Autodesk Inventor part; units mm, degrees
ref_plane "YZ Plane" through (0, 0, 0) normal (1, 0, 0) x (0, 1, 0)
ref_plane "XZ Plane" through (0, 0, 0) normal (0, 1, 0) x (-1, 0, 0)
ref_plane "XY Plane" through (0, 0, 0) normal (0, 0, 1) x (1, 0, 0)
sketch "Sketch1" plane through (0, 0, 0) normal (0, 0, 1) x (1, 0, 0)
  line L0 (19.1414, -92.5) -> (-27.8586, -92.5) construction
  line L1 (0, 3) -> (19.1414, 3) construction
  line L2 (6.5333, -102.5) -> (6.5333, -92.5) construction
  line L3 (-26.1333, -92.5) -> (-26.1333, -102.5) construction
  line L4 (-26.1333, -92.5) -> (-20.6889, -92.5)
  line L5 (19.1414, 3) -> (-27.8586, 3)
  line L6 (-27.8586, 3) -> (-27.8586, -92.5)
  line L7 (-27.8586, -92.5) -> (-20.6889, -92.5)
  line L8 (19.1414, -92.5) -> (19.1414, 3)
  line L9 (-27.8586, 3) -> (19.1414, 3)
  line L10 (19.1414, 3) -> (19.1414, 8)
  line L11 (19.1414, 8) -> (-27.8586, 8)
  line L12 (-27.8586, 8) -> (-27.8586, 3)
  line L13 (-6.3, -92.5) -> (-6.3, -95.5)
  line L14 (-6.3, -95.5) -> (1.0889, -95.5)
  line L15 (1.0889, -95.5) -> (1.0889, -92.5)
  line L16 (-13.3, -92.5) -> (-13.3, -95.5)
  line L17 (-13.3, -95.5) -> (-20.6889, -95.5)
  line L18 (-20.6889, -95.5) -> (-20.6889, -92.5)
  line L19 (-8.3, -92.5) -> (-8.3, -90.5)
  line L20 (-8.3, -90.5) -> (-7.15, -90.5)
  line L21 (-7.15, -90.5) -> (-7.15, -88.1)
  line L22 (-7.15, -88.1) -> (-8.3, -88.1)
  line L23 (-8.3, -88.1) -> (-8.3, -87.5)
  line L24 (-8.3, -87.5) -> (-11.3, -87.5)
  line L25 (-11.3, -87.5) -> (-11.3, -88.1)
  line L26 (-11.3, -88.1) -> (-12.45, -88.1)
  line L27 (-12.45, -88.1) -> (-12.45, -90.5)
  line L28 (-12.45, -90.5) -> (-11.3, -90.5)
  line L29 (-11.3, -92.5) -> (-11.3, -90.5)
  line L30 (-8.3, -92.5) -> (-6.3, -92.5)
  line L31 (-13.3, -92.5) -> (-11.3, -92.5)
  line L32 (-9.8, -83.4221) -> (-9.8, -94.6081) construction
  line L33 (-13.3, -92.5) -> (-11.3, -92.5)
  line L34 (1.0889, -92.5) -> (19.1414, -92.5)
  dimension "d4" = 5
  dimension "d13" = 5.3
  dimension "d14" = 2.4
  dimension "d15" = 3
  dimension "d16" = 32.6667
  dimension "d18" = 5.4444
  dimension "d19" = 5.4444
  dimension "d20" = 21.7778
  dimension "d21" = 7
  dimension "d22" = 3
  dimension "d23" = 5
  dimension "d24" = 8
extrude "Extrusion1" add sketch "Sketch1" along normal blind 3
sketch "Sketch2" plane through (0, 0, 3) normal (0, 0, 1) x (1, 0, 0)
  line L0 (7.3914, 0) -> (-0.1086, 0)
  line L1 (7.3914, 0) -> (7.3914, 3)
  line L2 (-0.1086, 3) -> (7.3914, 3)
  line L3 (-0.1086, 0) -> (-0.1086, 3)
  line L4 (-8.6086, 0) -> (-15.7666, 0)
  line L5 (-8.6086, 0) -> (-8.6086, 3)
  line L6 (-15.7666, 3) -> (-8.6086, 3)
  line L7 (7.3914, -34.3) -> (-0.1086, -34.3)
  line L8 (7.3914, -34.3) -> (7.3914, -31.3)
  line L9 (-0.1086, -31.3) -> (7.3914, -31.3)
  line L10 (-0.1086, -34.3) -> (-0.1086, -31.3)
  line L11 (-8.6086, -34.3) -> (-15.7666, -34.3)
  line L12 (-8.6086, -34.3) -> (-8.6086, -31.3)
  line L13 (-15.7666, -31.3) -> (-8.6086, -31.3)
  line L14 (7.3914, -44.3) -> (-0.1086, -44.3)
  line L15 (7.3914, -44.3) -> (7.3914, -41.3)
  line L16 (-0.1086, -41.3) -> (7.3914, -41.3)
  line L17 (-0.1086, -44.3) -> (-0.1086, -41.3)
  line L18 (-8.6086, -44.3) -> (-15.7666, -44.3)
  line L19 (-8.6086, -44.3) -> (-8.6086, -41.3)
  line L20 (-15.7666, -41.3) -> (-8.6086, -41.3)
  line L21 (-0.1086, -80.5) -> (7.3914, -80.5)
  line L22 (7.3914, -80.5) -> (7.3914, -77.5)
  line L23 (-0.1086, -77.5) -> (7.3914, -77.5)
  line L24 (-0.1086, -80.5) -> (-0.1086, -77.5)
  line L25 (-15.7666, -80.5) -> (-8.6086, -80.5)
  line L26 (-8.6086, -80.5) -> (-8.6086, -77.5)
  line L27 (-15.7666, -77.5) -> (-8.6086, -77.5)
  line L28 (-15.7666, -80.5) -> (-15.7666, -77.5)
  line L29 (-0.1086, 0) -> (-8.6086, 3) construction
  line L30 (-8.6086, 0) -> (-0.1086, 3) construction
  line L31 (-8.6086, -34.3) -> (-0.1086, -31.3) construction
  line L32 (-0.1086, -34.3) -> (-8.6086, -31.3) construction
  line L33 (-8.6086, -44.3) -> (-0.1086, -41.3) construction
  line L34 (-0.1086, -44.3) -> (-8.6086, -41.3) construction
  circle A0 centre (-4.3586, 1.5) radius 1.35
  circle A1 centre (-4.3586, -32.8) radius 1.35
  circle A2 centre (-4.3586, -42.8) radius 1.35
  line L35 (-0.1086, -77.5) -> (-8.6086, -80.5) construction
  line L36 (-8.6086, -77.5) -> (-0.1086, -80.5) construction
  circle A3 centre (-4.3586, -79) radius 1.35
  line L37 (-15.7666, 0) -> (-15.7666, 3)
  line L38 (-15.7666, -44.3) -> (-15.7666, -41.3)
  line L39 (-15.7666, -34.3) -> (-15.7666, -31.3)
  point P0 (0, 0)
  dimension "d5" = 2.7
  dimension "d6" = 2.7
  dimension "d7" = 2.7
  dimension "d8" = 2.7
extrude "Extrusion2" cut sketch "Sketch2" against normal blind 3
equation "\"d18\" = 0.166667 * d16"
equation "\"d19\" = d18"
CAD build for the part. Positions are in the model's coordinates, mm. A direction names the side the tool comes from. Give positions to 0.01 mm unless a question says otherwise; leave off trailing zeros. Loops run counter-clockwise (first coordinate to the right, second up) from the corner with the lowest first, then second, coordinate; pieces in that order, holes last. Notation, with made-up numbers: M 57,81 L 70,81 A14 cw 70,103 Z; hole C -30,17.25 d3. An arc over 180 degrees is marked long. One line per question, with ' | ' between items. Start each with the question number.
1. Saw through at A-A on y = -42.8. Give the cut face in (x, z).
2. Two-plate mould, pull along Y, no slides. Class faces 4 (the face through (-8.3, -92, 1)), 5 (the face through (-8.609, -33, 2)), 6 (the face through (-7, -92.5, 1)): pulls with the +Y half, pulls with the -Y half, needs draft (parallel to the pull), parting line crosses it, or undercut.
3. Flat gauge pin, fed straight in: pin 1 (1.5 mm diameter, centred on x = 12.5, z = 1, fed in from -Y). Where does the tip first touch, or does it go through?
4. Saw through at B-B on x = -4. Give the cut face in (y, z).
5. 3-axis set-ups, long thin cutter, end or side, ignore diameter. For faces 1 (the face through (4, -77.5, 2)), 2 (the face through (-11.3, -92, 1)), 3 (the face through (-17, -95.5, 1)): which of +Z, -Z, +X, -X, +Y, -Y reach the whole face in a straight line?
6. Probe L1, parallel to Y at x = -14.5, z = 0.85; L2, parallel to Y at x = -12.5, z = 2.9; L3, parallel to X at y = -79, z = 1.15. List the from-to ranges inside material, lowest first. Write a range as from..to.
7. Saw through at D-D on x = -25. Give the cut face in (y, z).
8. Saw through at C-C on z = 0.6. State how many separate pieces and enclosed holes the cut face has, plus the area to 3 significant figures.
Result sheet:
1) outline: M -27.86,0 L -15.77,0 L -15.77,3 L -27.86,3 Z; M -8.61,0 L -5.71,0 L -5.71,3 L -8.61,3 Z; M -3.01,0 L -0.11,0 L -0.11,3 L -3.01,3 Z; M 7.39,0 L 19.14,0 L 19.14,3 L 7.39,3 Z
2) face 4: needs draft | face 5: undercut | face 6: pulls with the -Y half
3) pin 1: stops at y = -92.5
4) outline: M -95.5,0 L -80.3,0 L -80.3,3 L -95.5,3 Z; M -77.7,0 L -44.1,0 L -44.1,3 L -77.7,3 Z; M -41.5,0 L -34.1,0 L -34.1,3 L -41.5,3 Z; M -31.5,0 L 0.2,0 L 0.2,3 L -31.5,3 Z; M 2.8,0 L 8,0 L 8,3 L 2.8,3 Z
5) face 1: +Z, -Z | face 2: +Z, -Z, -Y | face 3: +Z, -Z, +X, -X, -Y
6) L1: y = -95.5..-80.5, -77.5..-44.3, -41.3..-34.3, -31.3..0, 3..8 | L2: y = -92.5..-80.5, -77.5..-44.3, -41.3..-34.3, -31.3..0, 3..8 | L3: x = -27.86..-15.77, -8.61..-5.71, -3.01..-0.11, 7.39..19.14
7) outline: M -92.5,0 L 8,0 L 8,3 L -92.5,3 Z
8) separate pieces: 1 | enclosed holes: 12 | area: 4,550 mm^2
